Autodesk Inventor part; units mm, degrees
ref_plane "YZ Plane" through (0, 0, 0) normal (1, 0, 0) x (0, 1, 0)
ref_plane "XZ Plane" through (0, 0, 0) normal (0, 1, 0) x (-1, 0, 0)
ref_plane "XY Plane" through (0, 0, 0) normal (0, 0, 1) x (1, 0, 0)
sketch "Sketch1" plane through (0, 0, 0) normal (0, 0, 1) x (1, 0, 0)
  circle A0 centre (0, 0) radius 1.7526
  dimension "d0" = 3.5052
extrude "Extrusion1" add sketch "Sketch1" along normal blind 39.243
sketch "Sketch2" plane through (0, 0, 0) normal (0, 0, -1) x (-1, 0, 0)
  circle A0 centre (0, 0) radius 1.7526 construction
  circle A1 centre (0, 0) radius 2.8702
  dimension "d3" = 5.7404
extrude "Extrusion2" add sketch "Sketch2" along normal blind 3.5052
sketch "Sketch3" plane through (0, 0, -3.5052) normal (0, 0, -1) x (-1, 0, 0)
  circle A0 centre (0, 0) radius 2.8702
  line L0 (0, 1.604) -> (1.3891, 0.802)
  line L1 (1.3891, 0.802) -> (1.3891, -0.802)
  line L2 (1.3891, -0.802) -> (0, -1.604)
  line L3 (0, -1.604) -> (-1.3891, -0.802)
  line L4 (-1.3891, -0.802) -> (-1.3891, 0.802)
  line L5 (-1.3891, 0.802) -> (0, 1.604)
  dimension "d6" = 2.7781
extrude "Extrusion3" cut sketch "Sketch3" against normal blind 1.7526 contours L0 L1 L2 L3 L4 L5
chamfer "Chamfer1" distance 0.508 angle 45 1 edges at (-1.7526, 0, 39.243)
thread "Thread2"
properties part number "6-32 SHCS x1750 - .205" material "Stainless Steel"
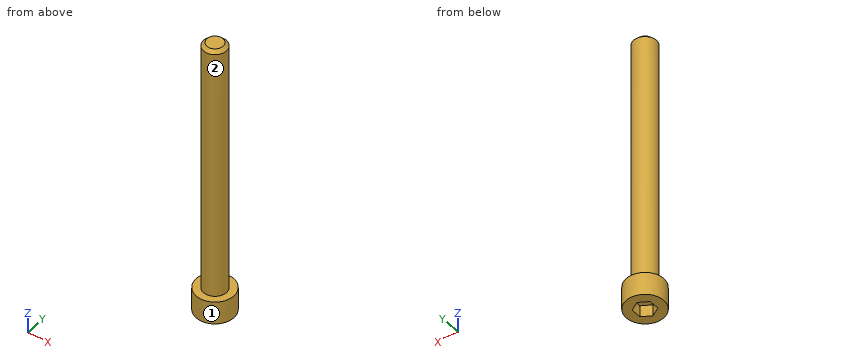
Can you work these out from the model? Positions are in its coordinate system, mm. Face numbers are marked on the shaded views. A direction names the side the tool comes from. Coordinates: 2 decimals unless noted, no trailing zeros. Loops run counter-clockwise (first coordinate to the right, second up) from the corner with the lowest first, then second, coordinate; pieces in that order, holes last. Notation, with made-up numbers: M -2.5,18.25 L 54.5,18.25 A24 cw 54.5,34.25 Z; hole C 47,49.25 d8. An arc over 180 degrees is marked long. Answer as CSV lines item,"result". Start each with the question number.
1. Suppose I cut it at A-A, the plane y = 0. List the corners of the cut face in (x, z) for me (3 decimals).
2. Suppose I cut it at B-B, the plane z = 3. List the corners of the cut face in (x, y) for me, plus the area to 3 significant figures.
3. For pin 1 Ø2 at (y, z) = (-1.5, 11) entering from +X; pin 2 Ø1.4 at (x, y) = (0.5, 0) entering from -Z; pin 3 Ø1 at (x, y) = (-0.5, 2) entering from +Z, each with a flat end and sliding along its axis, tell me the tip position at first contact or that it passes through.
4. For the marked faces 1 and 2, which set-ups out of +Z, -Z, +X, -X, +Y, -Y let a thin tool reach every point of the face, with its end or its side?
5. If I drill on probe 1 along X at (y, z) = (0.05, 13.5); probe 2 along Z at (x, y) = (-0.45, -2.35); probe 3 along Y at (x, z) = (0.7, 14), over which ranges is the centre line in solid material (lowest first)? Write a range as [from, to].
6. Suppose I cut it at C-C, the plane x = -2.4. List the corners of the cut face in (y, z) for me.
Output:
1,outline,"M -2.87,-3.505 L -1.389,-3.505 L -1.389,-1.753 L 1.389,-1.753 L 1.389,-3.505 L 2.87,-3.505 L 2.87,0 L 1.753,0 L 1.753,38.735 L 1.245,39.243 L -1.245,39.243 L -1.753,38.735 L -1.753,0 L -2.87,0 Z"
2,outline,"C 0,0 d3.51"
2,area,"9.65 mm^2"
3,pin 1,"stops at x = 1.68"
3,pin 2,"stops at z = -1.75"
3,pin 3,"stops at z = 38.93"
4,face 1,"+Z, -Z"
4,face 2,"+Z"
5,probe 1,"x = [-1.75, 1.75]"
5,probe 2,"z = [-3.51, 0]"
5,probe 3,"y = [-1.61, 1.61]"
6,outline,"M -1.57,-3.51 L 1.57,-3.51 L 1.57,0 L -1.57,0 Z"
